```python
from build123d import *

# Parameters (mm, degrees)
BOSS_EXTRUDE1_DEPTH  = 3.302
BOSS_EXTRUDE2_DEPTH  = 38.1
M5_CLEARANCE_HOLE1_D = 5.5
SKETCH6_W            = 199.898
SKETCH6_H            = 3.302
BOSS_EXTRUDE3_DEPTH  = 1.62
SKETCH7_W            = 199.898
SKETCH7_H            = 3.302
BOSS_EXTRUDE4_DEPTH  = 5.18


with BuildPart() as part:
    # Sketch1 → Boss-Extrude1 (new body)
    with BuildSketch(Plane(origin=(0, 0, 0), x_dir=(1, 0, 0), z_dir=(0, 1, 0))):
        Polygon((99.949, -81.28), (99.949, 101.6), (-99.949, 101.6), (-99.949, -81.28), (-79.629, -81.28), (-79.629, -101.6), (79.629, -101.6), (79.629, -81.28), align=None)
    extrude(amount=BOSS_EXTRUDE1_DEPTH)

    # Sketch3 → Boss-Extrude2 (add)
    with BuildSketch(Plane(origin=(0, 3.302, 0), x_dir=(1, 0, 0), z_dir=(0, 1, 0))):
        with BuildLine():
            Line((92.71, 48.26), (92.71, -27.94))
            ThreePointArc((92.71, -27.94), (86.36, -34.29), (80.01, -27.94))
            Line((80.01, -27.94), (80.01, 48.26))
            ThreePointArc((80.01, 48.26), (86.36, 54.61), (92.71, 48.26))
        make_face()
        with BuildLine():
            Line((-80.01, 48.26), (-80.01, -27.94))
            ThreePointArc((-80.01, -27.94), (-86.36, -34.29), (-92.71, -27.94))
            Line((-92.71, -27.94), (-92.71, 48.26))
            ThreePointArc((-92.71, 48.26), (-86.36, 54.61), (-80.01, 48.26))
        make_face()
    extrude(amount=BOSS_EXTRUDE2_DEPTH)

    # M5 Clearance Hole1 (through all)
    with Locations(Plane(origin=(0, 3.302, 0), x_dir=(1, 0, 0), z_dir=(0, 1, 0))):
        with Locations((-89.789, -55.88), (-89.789, 76.2), (89.789, -55.88), (89.789, 76.2)):
            Hole(M5_CLEARANCE_HOLE1_D / 2)

    # Sketch6 → Boss-Extrude3 (add)
    with BuildSketch(Plane(origin=(0, 0, -101.6), x_dir=(-1, 0, 0), z_dir=(0, 0, -1))):
        with Locations((0, 1.651)):
            Rectangle(SKETCH6_W, SKETCH6_H)
    extrude(amount=BOSS_EXTRUDE3_DEPTH)

    # Sketch7 → Boss-Extrude4 (add)
    with BuildSketch(Plane(origin=(0, 0, -103.22), x_dir=(-1, 0, 0), z_dir=(0, 0, -1))):
        with Locations((0, 1.651)):
            Rectangle(SKETCH7_W, SKETCH7_H)
    extrude(amount=BOSS_EXTRUDE4_DEPTH)


solid = part.part
```
Input: part model. Units: mm. Frame: model coordinates. A direction names the side the tool comes from. Coordinates: 2 decimals unless noted, no trailing zeros. Loops run counter-clockwise (first coordinate to the right, second up) from the corner with the lowest first, then second, coordinate; pieces in that order, holes last. Notation, with made-up numbers: (10, -24.5) -> (42, -24.5) arc R22 cw to (42, 0.5) -> close; hole circle Ø7 at (30.25, 12). An arc over 180 degrees is marked (long way). Use a Markdown table: item, result.
1) Cut plane D-D (x = -84). Return the cut outline in (y, z).
Results found:
| item | result |
|---|---|
| outline | (0, -108.4) -> (3.3, -108.4) -> (3.3, -54.16) -> (41.4, -54.16) -> (41.4, 33.84) -> (3.3, 33.84) -> (3.3, 81.28) -> (0, 81.28) -> close |
2) Cut plane B-B (z = 55.88). Return the cut outline in (x, y).
Results found:
| item | result |
|---|---|
| outline | (-99.95, 0) -> (-92.54, 0) -> (-92.54, 3.3) -> (-99.95, 3.3) -> close; (-87.04, 0) -> (87.04, 0) -> (87.04, 3.3) -> (-87.04, 3.3) -> close; (92.54, 0) -> (99.95, 0) -> (99.95, 3.3) -> (92.54, 3.3) -> close |
3) Contact query for flat-ended pins moving along their axis: pin 1 (9 mm diameter, centred on x = -89.789, z = -76.2, fed in from +Y); pin 2 (1 mm diameter, centred on y = 32.5, z = -14.5, fed in from -X); pin 3 (10 mm diameter, centred on x = 72.5, y = 14.5, fed in from -Z); pin 4 (3.5 mm diameter, centred on y = 1.5, z = 89.5, fed in from +X). Output: stop coordinate, or through.
Results found:
| item | result |
|---|---|
| pin 1 | stops at y = 3.3 |
| pin 2 | stops at x = -92.71 |
| pin 3 | passes through |
| pin 4 | stops at x = 79.63 |
4) Material intervals for line 1 along X through (y, z) = (1, -76); line 2 along X through (y, z) = (2, 55); line 3 along Y through (x, z) = (26.5, 74.5), sorted ascending. Write a range as from..to.
Results found:
| item | result |
|---|---|
| line 1 | x = -99.95..-92.53, -87.05..87.05, 92.53..99.95 |
| line 2 | x = -99.95..-92.39, -87.18..87.18, 92.39..99.95 |
| line 3 | y = 0..3.3 |
5) Pull-direction query (X, two-part tool) for faces 1 (the flat face through (92.71, 22, -11)), 2 (the flat face through (-86, 41.402, -11)), 3 (the cylindrical face through (86.5, 22.09, 34.29)), 4 (the flat face through (-92.71, 22, -10)); classes: released by +X, released by -X, zero draft, split by the parting line, or undercut.
Results found:
| item | result |
|---|---|
| face 1 | released by +X |
| face 2 | zero draft |
| face 3 | undercut |
| face 4 | released by -X |
6) Access query for faces 5 (the cylindrical face through (-87.04, 1.63, -76.32)), 6 (the cylindrical face through (-86.5, 22.09, -54.61)), 7 (the flat face through (80.01, 22, -10)), 8 (the cylindrical face through (-86.22, 22.09, 34.29)). Directions: +Z, -Z, +X, -X, +Y, -Y. A direction counts if a zero-diameter tool reaches every point of the face in a straight line with its end or side. Return the directions, or none.
Results found:
| item | result |
|---|---|
| face 5 | +Y, -Y |
| face 6 | -Z, +Y |
| face 7 | +Z, -Z, +Y |
| face 8 | +Z, +Y |
7) Cut plane C-C (z = 3). Return the cut outline in (x, y).
Results found:
| item | result |
|---|---|
| outline | (-99.95, 0) -> (99.95, 0) -> (99.95, 3.3) -> (92.71, 3.3) -> (92.71, 41.4) -> (80.01, 41.4) -> (80.01, 3.3) -> (-80.01, 3.3) -> (-80.01, 41.4) -> (-92.71, 41.4) -> (-92.71, 3.3) -> (-99.95, 3.3) -> close |
8) Cut plane A-A (y = 27). Return the cut outline in (x, z).
Results found:
| item | result |
|---|---|
| outline | (-92.71, -48.26) arc R6.35 ccw to (-80.01, -48.26) -> (-80.01, 27.94) arc R6.35 ccw to (-92.71, 27.94) -> close; (80.01, -48.26) arc R6.35 ccw to (92.71, -48.26) -> (92.71, 27.94) arc R6.35 ccw to (80.01, 27.94) -> close |
